Source: CAD feature listing. Evaluate the final solid. Frame: model axes, mm. A direction names the side the tool comes from. Give positions to 0.01 mm unless a question says otherwise; leave off trailing zeros. Loops run counter-clockwise (first coordinate to the right, second up) from the corner with the lowest first, then second, coordinate; pieces in that order, holes last. Notation, with made-up numbers: M 19.25,-9.75 L 24.25,-9.75 A25 ccw 24.25,12.25 Z; hole C 19,39.25 d6. An arc over 180 degrees is marked long. Write item = value, one per line.
from build123d import *

# Parameters (mm, degrees)
SKETCH1_R                        = 48
SKETCH1_R_2                      = 8
EX_CARRIER_FRONT_PLATE_4MM_DEPTH = 3
SKETCH2_R                        = 6
CUT_PIN_HOLE_12_DEPTH            = 69.14690015
PAT_PIN_HOLES_3X120_COUNT        = 3
CUT_EXTRUDE1_DEPTH               = 1
SKETCH4_R                        = 15
SKETCH4_R_2                      = 2.75
CUT_EXTRUDE2_DEPTH               = 68.948509917
SKETCH5_R                        = 15
SKETCH5_R_2                      = 2.75
CUT_EXTRUDE3_DEPTH               = 68.948509917
SKETCH6_R                        = 2.75
CUT_EXTRUDE4_DEPTH               = 68.948509917
SKETCH7_R                        = 2.75
CUT_EXTRUDE5_DEPTH               = 68.948509917
SKETCH8_R                        = 5
CUT_EXTRUDE7_DEPTH               = 3.5


with BuildPart() as part:
    # Sketch1 → EX_Carrier_Front_Plate_4mm (new, symmetric)
    with BuildSketch(Plane.XY):
        Circle(SKETCH1_R)
        Circle(SKETCH1_R_2, mode=Mode.SUBTRACT)
    extrude(amount=EX_CARRIER_FRONT_PLATE_4MM_DEPTH, both=True)

    # Sketch2 → CUT_Pin_Hole__12 (cut, symmetric)
    with BuildSketch(Plane.XY.offset(3)):
        with Locations((0, 33.75)):
            Circle(SKETCH2_R)
    cut_pin_hole_12 = extrude(amount=CUT_PIN_HOLE_12_DEPTH, both=True, mode=Mode.SUBTRACT)

    # PAT_Pin_Holes_3x120: CUT_Pin_Hole__12 ×3 about axis
    pat_pin_holes_3x120_axis = Axis((0, 0, 0), (0, 0, 1))
    for i in range(1, PAT_PIN_HOLES_3X120_COUNT):
        add(cut_pin_hole_12.rotate(pat_pin_holes_3x120_axis, i * 360 / PAT_PIN_HOLES_3X120_COUNT), mode=Mode.SUBTRACT)

    # Sketch3 → Cut-Extrude1 (cut, symmetric)
    with BuildSketch(Plane(origin=(0, 0, 0), x_dir=(0, 0, -1), z_dir=(1, 0, 0))):
        Polygon((0, 48), (-3, 44.889253006), (-3, 48), align=None)
    extrude(amount=CUT_EXTRUDE1_DEPTH, both=True, mode=Mode.SUBTRACT)

    # Sketch4 → Cut-Extrude2 (cut, through all)
    with BuildSketch(Plane.XY):
        Circle(SKETCH4_R)
        with Locations((0, -33.75)):
            Circle(SKETCH4_R_2)
    extrude(amount=CUT_EXTRUDE2_DEPTH, mode=Mode.SUBTRACT)

    # Sketch5 → Cut-Extrude3 (cut, through all)
    with BuildSketch(Plane.XY):
        Circle(SKETCH5_R)
        with Locations((0, -33.75)):
            Circle(SKETCH5_R_2)
    extrude(amount=-CUT_EXTRUDE3_DEPTH, mode=Mode.SUBTRACT)

    # Sketch6 → Cut-Extrude4 (cut, through all)
    with BuildSketch(Plane.XY):
        with Locations((29.228, 16.875)):
            Circle(SKETCH6_R)
        with Locations((-29.228, 16.875)):
            Circle(SKETCH6_R)
    extrude(amount=CUT_EXTRUDE4_DEPTH, mode=Mode.SUBTRACT)

    # Sketch7 → Cut-Extrude5 (cut, through all)
    with BuildSketch(Plane.XY):
        with Locations((29.228, 16.875)):
            Circle(SKETCH7_R)
        with Locations((-29.228, 16.875)):
            Circle(SKETCH7_R)
    extrude(amount=-CUT_EXTRUDE5_DEPTH, mode=Mode.SUBTRACT)

    # Sketch8 → Cut-Extrude7 (cut)
    with BuildSketch(Plane.XY.offset(3)):
        with Locations((0, -33.75)):
            Circle(SKETCH8_R)
        with Locations((29.228, 16.875)):
            Circle(SKETCH8_R)
        with Locations((-29.228, 16.875)):
            Circle(SKETCH8_R)
    extrude(amount=-CUT_EXTRUDE7_DEPTH, mode=Mode.SUBTRACT)


solid = part.part
1. Cut plane A-A, the plane y = 0. Return the cut outline in (x, z).
Derived:
outline = M -48,-3 L -15,-3 L -15,3 L -48,3 Z; M 15,-3 L 48,-3 L 48,3 L 15,3 Z
2. First-contact query: pin 1 Ø9 at (x, y) = (29.228, 16.875) entering from +Z; pin 2 Ø3 at (y, z) = (-20, -2) entering from +X; pin 3 Ø2 at (x, z) = (2, -2) entering from -Y. Flat tips, straight axial feed; report the tip coordinate or a pass-through.
Derived:
pin_1 = -0.5
pin_2 = 44.29
pin_3 = -47.99
3. Cut plane C-C, the plane z = 1.15. Return the cut outline in (x, y) (3 decimals).
Derived:
outline = M -1,46.808 L -1,47.99 A48 ccw long 1,47.99 L 1,46.808 Z; hole C -29.228,-16.875 d12; hole C -29.228,16.875 d10; hole C 0,0 d30; hole C 0,33.75 d12; hole C 0,-33.75 d10; hole C 29.228,-16.875 d12; hole C 29.228,16.875 d10
4. Material intervals for probe 1 along Y at (x, z) = (0, -1.3); probe 2 along Y at (x, z) = (-25.5, 2.7); probe 3 along Y at (x, z) = (5.5, -0.45), sorted ascending. Write a range as from..to.
Derived:
probe_1 = -48..-36.5, -31..-15, 15..27.75, 39.75..48
probe_2 = -40.67..-21.58, -12.17..13.54, 20.21..40.67
probe_3 = -47.68..-13.96, 13.96..31.35, 36.15..47.68
5. Pull-direction query (X, two-part tool) for faces 1 (the cylindrical face through (-30.312, 11.994, 1.274)), 2 (the cylindrical face through (-47.954, 2.11, 0.042)), 3 (the flat face through (-11, 11, -3)), 4 (the cylindrical face through (28.87, 19.6, -1.73)); classes: +X half, -X half, draft (parallel to the pull), parting line (faces both ways), or undercut.
Derived:
face_1 = undercut
face_2 = parting line
face_3 = draft
face_4 = undercut
6. Cut plane B-B, the plane x = 12. Return the cut outline in (y, z), then the cut area to 3 significant figures.
Derived:
outline = M -46.48,-3 L -9,-3 L -9,3 L -46.48,3 Z; M 9,-3 L 46.48,-3 L 46.48,3 L 9,3 Z
area = 450 mm²
7. Reachability of faces 5 (the flat face through (2, -36, -0.5)), 6 (the cylindrical face through (0, -31, -2)), 7 (the flat face through (0.014, 46.466, 1.479)) from +Z, -Z, +X, -X, +Y, -Y: full face, straight path, thin tool, end or side. Return the list, or none.
Derived:
face_5 = +Z
face_6 = +Z, -Z
face_7 = +Z, +Y
8. Cut plane D-D, the plane y = -20.5. Return the cut outline in (x, z), then the cut area to 3 significant figures.
Derived:
outline = M -43.4,-3 L -34.01,-3 L -34.01,3 L -43.4,3 Z; M -24.45,-3 L 24.45,-3 L 24.45,3 L -24.45,3 Z; M 34.01,-3 L 43.4,-3 L 43.4,3 L 34.01,3 Z
area = 406 mm²
